Part print with two shaded views. Sizes in mm from the minimum x, y, z corner. A direction names the side the tool comes from. Give positions to 0.01 mm unless a question says otherwise; leave off trailing zeros. Write each loop counter-clockwise with the first axis right and the second up, starting at its lowest first coordinate (ties: lowest second). Pieces come first, ordered by that corner, then holes. Notation, with made-up numbers: M 32,75 L 44,75 A8 cw 44,84 Z; hole C 86.25,-8.75 d2. An arc over 180 degrees is marked long. Return JSON: item names as keys, results as strings. Group by question number.
Q1. Flat gauge pins, fed straight in: pin 1 Ø5 at (y, z) = (20, 290.5) entering from +X; pin 2 Ø10.5 at (x, y) = (191, 19.5) entering from -Z; pin 3 Ø9 at (y, z) = (13, 11.5) entering from +X. Where does each tip first touch, or does it go through?
Q2. Pull direction X, two halves, no side cores. Call the marked faces 3, 4, 5 and 6: +X half, -X half, draft (parallel to the pull), parting line (faces both ways), or undercut.
Q3. Band-saw the part on B-B, the plane y = 19.5. Give the cut face in (x, z) (1 decimal).
Q4. Tool access for the marked faces 1 and 2: list every direction of +Z, -Z, +X, -X, +Y, -Y with a clear straight run to the whole face (end or side of a thin tool).
Q5. Wall check: probe 1 along Z at (x, y) = (60.5, 22); probe 2 along Z at (x, y) = (165, 18.5); probe 3 along X at (y, z) = (5, 224) (1 decimal). Give the ranges that are in metal, low to high.
Q6. Band-saw the part on A-A, the plane x = 63.5. Give the cut face in (y, z), then the cut area to 3 significant figures.
Q7. Band-saw the part on C-C, the plane z = 179. Give the cut face in (x, y) (1 decimal), then the cut area to 3 significant figures.
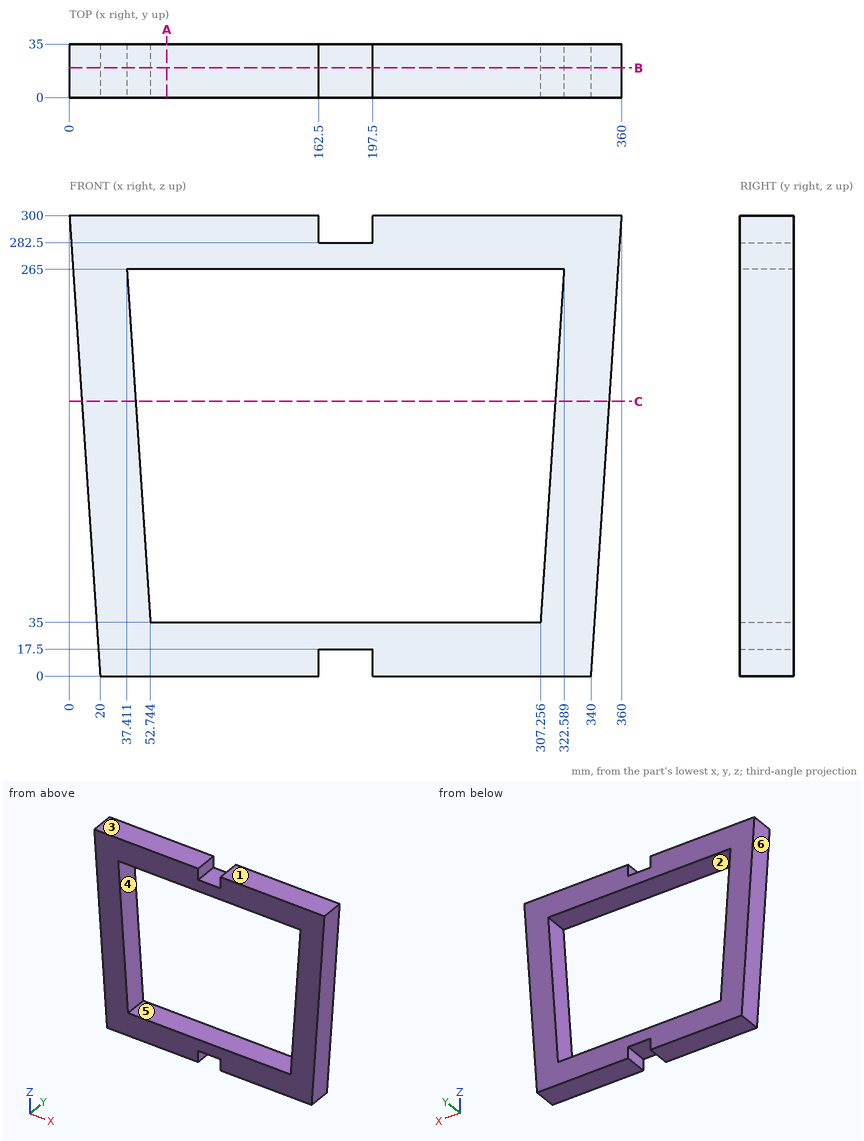
From the geometry:
{
 "1": {"pin 1": "stops at x = 359.53", "pin 2": "stops at z = 17.5", "pin 3": "stops at x = 341.07"},
 "2": {"face 3": "draft", "face 4": "undercut", "face 5": "undercut", "face 6": "-X half"},
 "3": {"outline": "M 0,300 L 20,0 L 162.5,0 L 162.5,17.5 L 197.5,17.5 L 197.5,0 L 340,0 L 360,300 L 197.5,300 L 197.5,282.5 L 162.5,282.5 L 162.5,300 Z; hole M 37.4,265 L 52.7,35 L 307.3,35 L 322.6,265 Z"},
 "4": {"face 1": "+Z, +X, -X, +Y, -Y", "face 2": "+Y, -Y"},
 "5": {"probe 1": "z = 0 to 35, 265 to 300", "probe 2": "z = 17.5 to 35, 265 to 282.5", "probe 3": "x = 5.1 to 40.1, 319.9 to 354.9"},
 "6": {"outline": "M 0,0 L 35,0 L 35,35 L 0,35 Z; M 0,265 L 35,265 L 35,300 L 0,300 Z", "area": "2,450 mm^2"},
 "7": {"outline": "M 8.1,0 L 43.1,0 L 43.1,35 L 8.1,35 Z; M 316.9,0 L 351.9,0 L 351.9,35 L 316.9,35 Z", "area": "2,460 mm^2"}
}
